Build history of the part. All positions in model axes, mm. Give positions to 0.01 mm unless a question says otherwise; leave off trailing zeros. Loops run counter-clockwise (first coordinate to the right, second up) from the corner with the lowest first, then second, coordinate; pieces in that order, holes last. Notation, with made-up numbers: M -26.75,-39 L 14.25,-39 A17 ccw 14.25,-11 Z; hole C -15,76 d8. An arc over 180 degrees is marked long. Put each result on its own line as item: value.
```python
from build123d import *

# Parameters (mm, degrees)
CYLINDER096_R           = 2
CYLINDER096_DEPTH       = 10
CYLINDER096_ROLL_ANGLE  = 90
CYLINDER097_R           = 2
CYLINDER097_DEPTH       = 10
CYLINDER097_ROLL_ANGLE  = 90
CYLINDER026_R           = 1.6
CYLINDER026_DEPTH       = 50
CYLINDER026_ROLL_ANGLE  = 90
CYLINDER025_R           = 1.6
CYLINDER025_DEPTH       = 50
CYLINDER025_ROLL_ANGLE  = 90
CYLINDER028_R           = 1.6
CYLINDER028_DEPTH       = 50
CYLINDER028_ROLL_ANGLE  = 90
CYLINDER027_R           = 1.6
CYLINDER027_DEPTH       = 50
CYLINDER027_ROLL_ANGLE  = 90
CYLINDER019_R           = 1.6
CYLINDER019_DEPTH       = 40
CYLINDER019_PITCH_ANGLE = 90
CYLINDER018_R           = 1.6
CYLINDER018_DEPTH       = 40
CYLINDER018_PITCH_ANGLE = 90
CYLINDER017_R           = 1.6
CYLINDER017_DEPTH       = 40
CYLINDER016_R           = 1.6
CYLINDER016_DEPTH       = 70
CYLINDER016_ROLL_ANGLE  = 90
CYLINDER015_R           = 1.6
CYLINDER015_DEPTH       = 40
BOX011_W                = 116
BOX011_H                = 5
BOX011_DEPTH            = 144


with BuildPart() as cylinder373:
    # Cylinder096 → Cylinder096 (new body)
    with BuildSketch(Plane.XY):
        Circle(CYLINDER096_R)
    extrude(amount=CYLINDER096_DEPTH)


with BuildPart() as cylinder373_1:
    # Cylinder096 roll: moved
    add(cylinder373.part.rotate(Axis((0, 0, 0), (1, 0, 0)), CYLINDER096_ROLL_ANGLE))


with BuildPart() as cylinder373_2:
    # Cylinder096 placement: moved
    add(cylinder373_1.part.moved(Location((-20, -15, 114))))


with BuildPart() as cylinder374:
    # Cylinder097 → Cylinder097 (new body)
    with BuildSketch(Plane.XY):
        Circle(CYLINDER097_R)
    extrude(amount=CYLINDER097_DEPTH)


with BuildPart() as cylinder374_1:
    # Cylinder097 roll: moved
    add(cylinder374.part.rotate(Axis((0, 0, 0), (1, 0, 0)), CYLINDER097_ROLL_ANGLE))


with BuildPart() as cylinder374_2:
    # Cylinder097 placement: moved
    add(cylinder374_1.part.moved(Location((64, -15, 16))))


with BuildPart() as cylinder033:
    # Cylinder026 → Cylinder026 (new body)
    with BuildSketch(Plane.XY):
        Circle(CYLINDER026_R)
    extrude(amount=CYLINDER026_DEPTH)


with BuildPart() as cylinder033_1:
    # Cylinder026 roll: moved
    add(cylinder033.part.rotate(Axis((0, 0, 0), (1, 0, 0)), CYLINDER026_ROLL_ANGLE))


with BuildPart() as cylinder033_2:
    # Cylinder026 placement: moved
    add(cylinder033_1.part.moved(Location((26.54, 7, 54))))


with BuildPart() as fusion031:
    # Cylinder025 → Cylinder025 (new body)
    with BuildSketch(Plane.XY):
        Circle(CYLINDER025_R)
    extrude(amount=CYLINDER025_DEPTH)


with BuildPart() as fusion031_1:
    # Cylinder025 roll: moved
    add(fusion031.part.rotate(Axis((0, 0, 0), (1, 0, 0)), CYLINDER025_ROLL_ANGLE))


with BuildPart() as fusion031_2:
    # Cylinder025 placement: moved
    add(fusion031_1.part.moved(Location((74.5, 7, 54))))

    # Fusion031: union Cylinder033
    add(cylinder033_2.part)


with BuildPart() as fusion032:
    # Cylinder028 → Cylinder028 (new body)
    with BuildSketch(Plane.XY):
        Circle(CYLINDER028_R)
    extrude(amount=CYLINDER028_DEPTH)


with BuildPart() as fusion032_1:
    # Cylinder028 roll: moved
    add(fusion032.part.rotate(Axis((0, 0, 0), (1, 0, 0)), CYLINDER028_ROLL_ANGLE))


with BuildPart() as fusion032_2:
    # Cylinder028 placement: moved
    add(fusion032_1.part.moved(Location((31, 7, 104.5))))

    # Fusion032: union Fusion031
    add(fusion031_2.part)


with BuildPart() as arduino_holes:
    # Cylinder027 → Cylinder027 (new body)
    with BuildSketch(Plane.XY):
        Circle(CYLINDER027_R)
    extrude(amount=CYLINDER027_DEPTH)


with BuildPart() as arduino_holes_1:
    # Cylinder027 roll: moved
    add(arduino_holes.part.rotate(Axis((0, 0, 0), (1, 0, 0)), CYLINDER027_ROLL_ANGLE))


with BuildPart() as arduino_holes_2:
    # Cylinder027 placement: moved
    add(arduino_holes_1.part.moved(Location((59, 7, 104.5))))

    # Fusion033: union Fusion032
    add(fusion032_2.part)


with BuildPart() as arduino_holes_3:
    # Fusion033 placement: moved
    add(arduino_holes_2.part.moved(Location((5, 0, 21))))


with BuildPart() as cylinder100:
    # Cylinder019 → Cylinder019 (new body)
    with BuildSketch(Plane.XY):
        Circle(CYLINDER019_R)
    extrude(amount=CYLINDER019_DEPTH)


with BuildPart() as cylinder100_1:
    # Cylinder019 pitch: moved
    add(cylinder100.part.rotate(Axis((0, 0, 0), (0, 1, 0)), CYLINDER019_PITCH_ANGLE))


with BuildPart() as cylinder100_2:
    # Cylinder019 placement: moved
    add(cylinder100_1.part.moved(Location((-40, 12, 9.5))))


with BuildPart() as fusion011:
    # Cylinder018 → Cylinder018 (new body)
    with BuildSketch(Plane.XY):
        Circle(CYLINDER018_R)
    extrude(amount=CYLINDER018_DEPTH)


with BuildPart() as fusion011_1:
    # Cylinder018 pitch: moved
    add(fusion011.part.rotate(Axis((0, 0, 0), (0, 1, 0)), CYLINDER018_PITCH_ANGLE))


with BuildPart() as fusion011_2:
    # Cylinder018 placement: moved
    add(fusion011_1.part.moved(Location((-40, -7, 2.5))))

    # Fusion011: union Cylinder100
    add(cylinder100_2.part)


with BuildPart() as fusion012:
    # Cylinder017 → Cylinder017 (new body)
    with BuildSketch(Plane(origin=(-27.5, 7, -15), x_dir=(1, 0, 0), z_dir=(0, 0, 1))):
        Circle(CYLINDER017_R)
    extrude(amount=CYLINDER017_DEPTH)

    # Fusion012: union Fusion011
    add(fusion011_2.part)


with BuildPart() as fusion013:
    # Cylinder016 → Cylinder016 (new body)
    with BuildSketch(Plane.XY):
        Circle(CYLINDER016_R)
    extrude(amount=CYLINDER016_DEPTH)


with BuildPart() as fusion013_1:
    # Cylinder016 roll: moved
    add(fusion013.part.rotate(Axis((0, 0, 0), (1, 0, 0)), CYLINDER016_ROLL_ANGLE))


with BuildPart() as fusion013_2:
    # Cylinder016 placement: moved
    add(fusion013_1.part.moved(Location((-24, 39, 6))))

    # Fusion013: union Fusion012
    add(fusion012.part)


with BuildPart() as cylinder008:
    # Cylinder015 → Cylinder015 (new body)
    with BuildSketch(Plane(origin=(-20.5, -12, -15), x_dir=(1, 0, 0), z_dir=(0, 0, 1))):
        Circle(CYLINDER015_R)
    extrude(amount=CYLINDER015_DEPTH)


with BuildPart() as face_corner_holes015:
    # Fusion029 base: copy of Cylinder008
    add(cylinder008.part)

    # Fusion029: union Fusion013
    add(fusion013_2.part)


with BuildPart() as face_corner_holes015_1:
    # Fusion029 placement: moved
    add(face_corner_holes015.part.moved(Location((104, 0, 132))))


with BuildPart() as face_corner_holes011:
    # Fusion025 base: copy of Cylinder008
    add(cylinder008.part)

    # Fusion025: union Fusion013
    add(fusion013_2.part)


with BuildPart() as face_corner_holes011_1:
    # Fusion025 placement: moved
    add(face_corner_holes011.part.moved(Location((0, 0, 132))))


with BuildPart() as face_corner_holes007:
    # Fusion021 base: copy of Cylinder008
    add(cylinder008.part)

    # Fusion021: union Fusion013
    add(fusion013_2.part)


with BuildPart() as face_corner_holes007_1:
    # Fusion021 placement: moved
    add(face_corner_holes007.part.moved(Location((104, 0, 0))))


with BuildPart() as face_corner_holes004:
    # Fusion018 base: copy of Cylinder008
    add(cylinder008.part)

    # Fusion018: union Fusion013
    add(fusion013_2.part)


with BuildPart() as back_a:
    # Box011 → Box011 (new body)
    with BuildSketch(Plane(origin=(-30, -23, 0), x_dir=(1, 0, 0), z_dir=(0, 0, 1))):
        with Locations((58, 2.5)):
            Rectangle(BOX011_W, BOX011_H)
    extrude(amount=BOX011_DEPTH)

    # Cut013: cut face-corner-holes004
    add(face_corner_holes004.part, mode=Mode.SUBTRACT)

    # Cut017: cut face-corner-holes007
    add(face_corner_holes007_1.part, mode=Mode.SUBTRACT)

    # Cut022: cut face-corner-holes011
    add(face_corner_holes011_1.part, mode=Mode.SUBTRACT)

    # Cut027: cut face-corner-holes015
    add(face_corner_holes015_1.part, mode=Mode.SUBTRACT)

    # Cut028: cut arduino-holes
    add(arduino_holes_3.part, mode=Mode.SUBTRACT)

    # Cut057: cut Cylinder374
    add(cylinder374_2.part, mode=Mode.SUBTRACT)

    # Cut058: cut Cylinder373
    add(cylinder373_2.part, mode=Mode.SUBTRACT)


solid = back_a.part
```
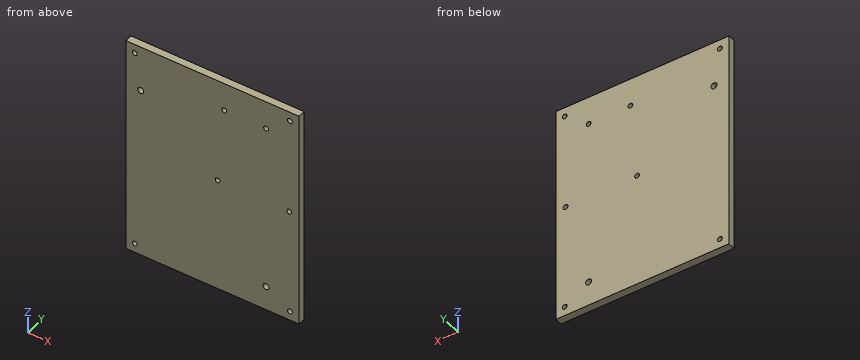
Q1. Slice it at A-A (z = 138). List the corners of the cut face in (x, y).
Here are the results:
outline: M -30,-23 L -25.6,-23 L -25.6,-18 L -30,-18 Z; M -22.4,-23 L 78.4,-23 L 78.4,-18 L -22.4,-18 Z; M 81.6,-23 L 86,-23 L 86,-18 L 81.6,-18 Z
Q2. Slice it at B-B (x = -24). List the corners of the cut face in (y, z), and give its area (3 significant figures).
Here are the results:
outline: M -23,0 L -18,0 L -18,4.4 L -23,4.4 Z; M -23,7.6 L -18,7.6 L -18,136.4 L -23,136.4 Z; M -23,139.6 L -18,139.6 L -18,144 L -23,144 Z
area: 688 mm²
Q3. Drop a flat-ended pin along its axis: pin 1 Ø2.5 at (x, z) = (79.5, 75) entering from -Y. Give the stop position or say it passes through.
Here are the results:
pin 1: through
Q4. Slice it at C-C (z = 114). List the corners of the cut face in (x, y).
Here are the results:
outline: M -30,-23 L -22,-23 L -22,-18 L -30,-18 Z; M -18,-23 L 86,-23 L 86,-18 L -18,-18 Z
Q5. Probe line 1 (Z direction, x = -24, y = -20.4); line 2 (X direction, y = -21.65, z = 125.5); line 3 (Z direction, x = 64, y = -20.45). List the from-to ranges inside material, lowest first. Write a range as from..to.
Here are the results:
line 1: 0..4.4, 7.6..136.4, 139.6..144
line 2: -30..34.4, 37.6..62.4, 65.6..86
line 3: 0..14, 18..123.9, 127.1..144
Q6. Slice it at D-D (x = 31.54). List the corners of the cut face in (y, z).
Here are the results:
outline: M -23,0 L -18,0 L -18,73.4 L -23,73.4 Z; M -23,76.6 L -18,76.6 L -18,144 L -23,144 Z
